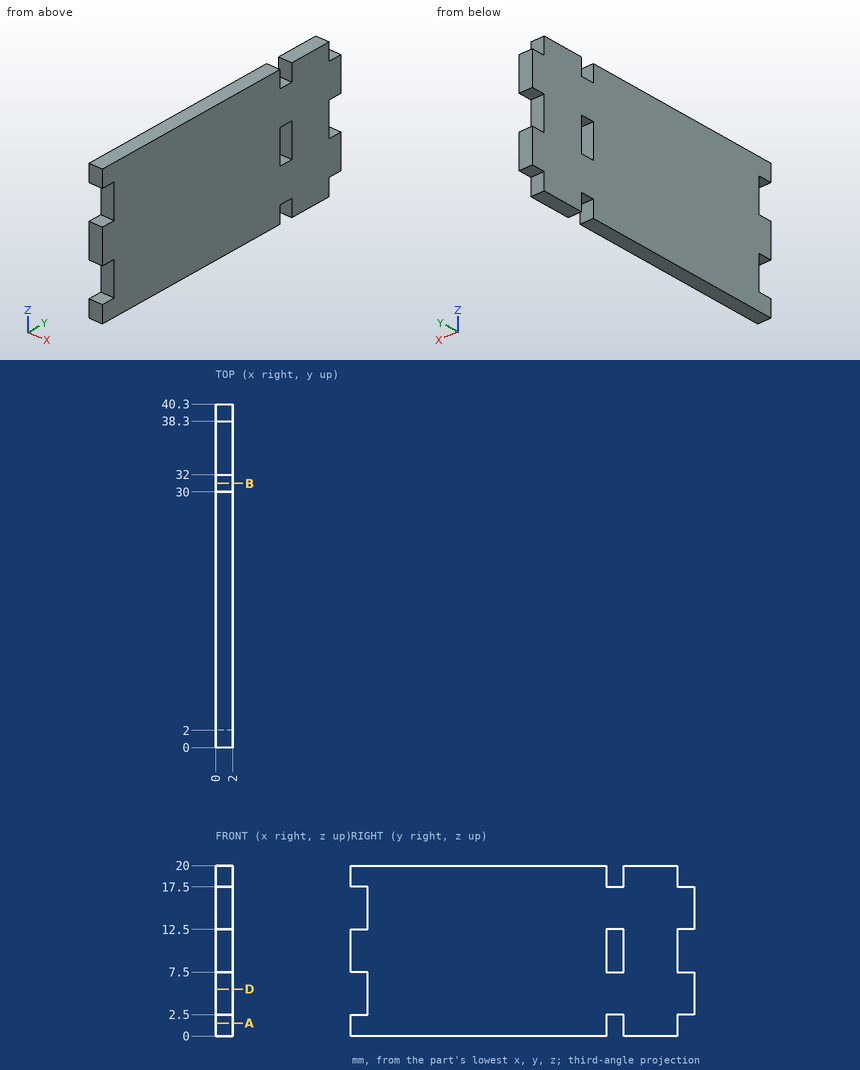
Job drawing, mm, ordinate dimensions from the low corner. One solid piece. Coordinates: 2 decimals unless noted, no trailing zeros. Write each loop counter-clockwise with the first axis right and the second up, starting at its lowest first coordinate (ties: lowest second). Pieces come first, ordered by that corner, then holes. Notation, with made-up numbers: M 2.5,-2 L 35.5,-2 A15 ccw 35.5,6 Z; hole C 46.25,53.25 d3. An arc over 180 degrees is marked long. Answer as a JSON object with one key per item and string values. Group by question number.
1) Saw through at A-A (z = 1.5). Write the cut outline in (x, y).
2) Saw through at D-D (z = 5.5). Write the cut outline in (x, y), plus the area to 3 significant figures.
3) Wall check: line 1 (Y direction, x = 1.05, z = 17.75); line 2 (Y direction, x = 1.9, z = 13.25). Give the ranges that are in metal, low to high. Write a range as from..to.
4) Pin check, flat tips, straight feed: pin 1 Ø0.6 at (x, z) = (0.5, 16) entering from -Y; pin 2 Ø1 at (x, y) = (1, 31) entering from -Z; pin 3 Ø1 at (x, y) = (1, 39) entering from +Z. Stop position of each tip, or through.
5) Saw through at B-B (y = 31). Write the cut outline in (x, z).
Values follow:
{
 "1": {"outline": "M 0,0 L 2,0 L 2,30 L 0,30 Z; M 0,32 L 2,32 L 2,38.3 L 0,38.3 Z"},
 "2": {"outline": "M 0,2 L 2,2 L 2,40.3 L 0,40.3 Z", "area": "76.6 mm2"},
 "3": {"line 1": "y = 0..30, 32..38.3", "line 2": "y = 2..40.3"},
 "4": {"pin 1": "stops at y = 2", "pin 2": "stops at z = 2.5", "pin 3": "stops at z = 17.5"},
 "5": {"outline": "M 0,2.5 L 2,2.5 L 2,7.5 L 0,7.5 Z; M 0,12.5 L 2,12.5 L 2,17.5 L 0,17.5 Z"}
}
